```python
from build123d import *

# Parameters (mm, degrees)
F1_DEPTH = 5
F2_R     = 2.5
F3_R     = 2.49999
F7_ANGLE = 180


# Not quite as in the source:
# - a fillet or chamfer is up to 0.001 mm smaller than in the source, because OpenCascade refuses the exact size


with BuildPart() as f1:
    # F0 (on Top) → F1 (new body)
    with BuildSketch(Plane.XY):
        Polygon((0, 72.5676417351), (0, 0), (187.6123100519, -13.9679014683), (187.6123100519, 26.09346807), align=None)
    extrude(amount=F1_DEPTH)

    # F2
    f2_edges = [f1.edges().sort_by_distance(p)[0] for p in [
        (93.806155, 49.330555, 5),
    ]]
    fillet(f2_edges, radius=F2_R)

    # F3 (radius 2.5 in the source; OpenCascade refuses exactly that, so slightly less here)
    f3_edges = [f1.edges().sort_by_distance(p)[0] for p in [
        (93.806155, 49.330555, 0),
    ]]
    fillet(f3_edges, radius=F3_R)


with BuildPart() as f4_1:
    # F4: instance of F1
    add(f1.part.mirror(Plane.YZ))


with BuildPart() as f1_1:
    add(f1.part)

    add(f4_1.part)  # F5 merges F4_1
    # F5: F1 across plane
    add(f1.part.mirror(Plane.YZ))


with BuildPart() as f1_2:
    # F7: moved
    add(f1_1.part.rotate(Axis((0, 0, 62.2569620609), (0, 0, 1)), F7_ANGLE))


solid = f1_2.part
```
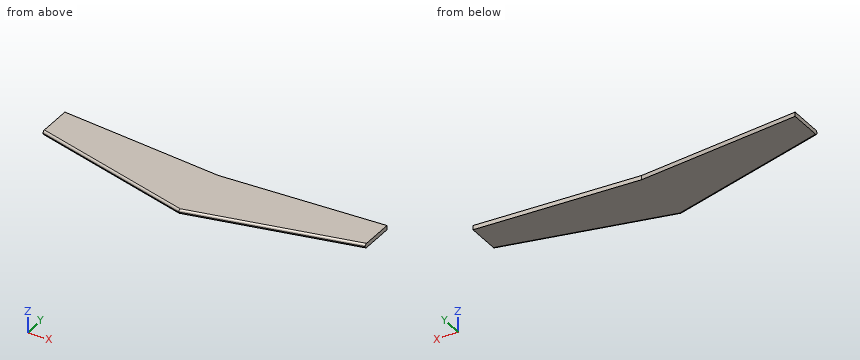
Work out the finished part from the listing and answer in its coordinate system (mm). Give positions to 0.01 mm unless a question says otherwise; leave off trailing zeros. Loops run counter-clockwise (first coordinate to the right, second up) from the corner with the lowest first, then second, coordinate; pieces in that order, holes last. Notation, with made-up numbers: (-9.75, 57.25) -> (7.25, 57.25) arc R31 ccw to (7.25, 93.25) -> close; hole circle Ø10 at (52, 76.5). An arc over 180 degrees is marked (long way). One line per question, with ' | ' between items. Start each with the question number.
1) This flat-tipped pin is pushed along its axis until it touches: pin 1 (1 mm diameter, centred on x = -77.5, z = 1, fed in from -Y). Where does it stop, or does it pass through?
2) Straight lines are drawn through the part: L1, parallel to Y at x = 143, z = 2; L2, parallel to Y at x = 48.5, z = 3.95. For each, find the intervals that lie inside material, in ascending order.
3) Section A-A, the plane z = 3.7 is taken. Determine the outline of the cut face in (x, y), then the cut area to 3 significant figures.
Resolved:
1) pin 1: y = -53.19
2) L1: -37.09 to 10.65 | L2: -60.08 to 3.61
3) outline: (-187.61, -25.78) -> (0, -72.25) -> (187.61, -25.78) -> (187.61, 13.97) -> (0, 0) -> (-187.61, 13.97) -> close | area: 21,000 mm2
